Input: part model. Units: mm. Frame: model coordinates. A direction names the side the tool comes from. Give positions to 0.01 mm unless a question says otherwise; leave off trailing zeros. Loops run counter-clockwise (first coordinate to the right, second up) from the corner with the lowest first, then second, coordinate; pieces in that order, holes last. Notation, with made-up numbers: M 89,35.25 L 118,35.25 A25 cw 118,55.25 Z; hole C 89.5,46.5 d11. An arc over 180 degrees is marked long. One line per item, written item: value. Start each with the question number.
(1) Section A-A on y = 1.85. State how many separate pieces and enclosed holes the cut face has, plus the area to 3 significant figures.
(2) Access query for faces 1 (the cylindrical face through (-1.2, 1.5, -8.6)), 2 (the flat face through (66.183, 1.479, 16.42)). Directions: +Z, -Z, +X, -X, +Y, -Y. A direction counts if a zero-diameter tool reaches every point of the face in a straight line with its end or side. Return the directions, or none.
(3) Ray query, line 1 along X through (y, z) = (1.9, 18); line 2 along X through (y, z) = (2, -3); line 3 along Z through (x, y) = (47, 1). Return the intervals inside material, ascending. Write a range as from..to.
(4) Pull-direction query (X, two-part tool) for faces 3 (the flat face through (-94, 1.5, 16.2)), 4 (the flat face through (93.85, 1.48, 16.38)), 5 (the cylindrical face through (-85.414, 1.521, -7.208)), 6 (the flat face through (-1, 3, -5)); classes: released by +X, released by -X, zero draft, split by the parting line, or undercut.
(5) Section B-B on x = -38. Output: boundary loops of the cut face in (y, z), plus the area to 3 significant figures.
```python
from build123d import *

# Parameters (mm, degrees)
SKETCH_1_W             = 200
SKETCH_1_H             = 48
EXTRUDE_1_DEPTH        = 3
SKETCH_2_R             = 2
CUT_EXTRUDE_1_DEPTH    = 3
SKETCH_3_R             = 10.5
CUT_EXTRUDE_2_DEPTH    = 0.1
SKETCH_5_R             = 2
SKETCH_5_R_2           = 1.6
CUT_EXTRUDE_3_DEPTH    = 10
SKETCH_7_W             = 200
SKETCH_7_H             = 1.5
CUT_EXTRUDE_4_DEPTH    = 10
SKETCH_9_R             = 10.5
SKETCH_9_R_2           = 1.6
SKETCH_9_R_3           = 2
EXTRUDE_3_DEPTH        = 0.1
CUT_EXTRUDE_3602_DEPTH = 10
SKETCH_11_W            = 11
SKETCH_11_H            = 7
CUT_EXTRUDE_6_DEPTH    = 10
FILLET_1_R             = 5
FILLET_2_R             = 5
FILLET_3_R             = 0.8


with BuildPart() as part:
    # 草图1 → 凸台-拉伸1 (new body)
    with BuildSketch(Plane(origin=(0, 0, 0), x_dir=(1, 0, 0), z_dir=(0, 1, 0))):
        Rectangle(SKETCH_1_W, SKETCH_1_H)
    extrude(amount=EXTRUDE_1_DEPTH)

    # 草图2 → 切除-拉伸1 (cut)
    with BuildSketch(Plane(origin=(0, 3, 0), x_dir=(1, 0, 0), z_dir=(0, 1, 0))):
        with Locations(Location((-80, -18, 0), (0, 0, 270))):
            Circle(SKETCH_2_R)
        with Locations(Location((0, -18, 0), (0, 0, 270))):
            Circle(SKETCH_2_R)
        with Locations(Location((80, -18, 0), (0, 0, 90))):
            Circle(SKETCH_2_R)
        with Locations(Location((-30, 15, 0), (0, 0, 270))):
            Circle(SKETCH_2_R)
        with Locations(Location((50, 15, 0), (0, 0, 270))):
            Circle(SKETCH_2_R)
    extrude(amount=-CUT_EXTRUDE_1_DEPTH, mode=Mode.SUBTRACT)

    # 草图3 → 切除-拉伸2 (cut)
    with BuildSketch(Plane(origin=(0, 3, 0), x_dir=(1, 0, 0), z_dir=(0, 1, 0))):
        with Locations(Location((-80, 7, 0), (0, 0, 270))):
            Circle(SKETCH_3_R)
        with Locations(Location((0, 7, 0), (0, 0, 270))):
            Circle(SKETCH_3_R)
        with Locations(Location((80, 7, 0), (0, 0, 90))):
            Circle(SKETCH_3_R)
    extrude(amount=-CUT_EXTRUDE_2_DEPTH, mode=Mode.SUBTRACT)

    # 草图5 → 切除-拉伸3 (cut)
    with BuildSketch(Plane(origin=(0, 3, 0), x_dir=(1, 0, 0), z_dir=(0, 1, 0))):
        with Locations(Location((0, 7, 0), (0, 0, 270))):
            Circle(SKETCH_5_R)
        with Locations(Location((0, 14, 0), (0, 0, 270))):
            Circle(SKETCH_5_R_2)
        with Locations(Location((-7, 7, 0), (0, 0, 270))):
            Circle(SKETCH_5_R_2)
        with Locations(Location((7, 7, 0), (0, 0, 270))):
            Circle(SKETCH_5_R_2)
        with Locations(Location((0, 0, 0), (0, 0, 270))):
            Circle(SKETCH_5_R_2)
        with Locations(Location((-80, 0, 0), (0, 0, 270))):
            Circle(SKETCH_5_R_2)
        with Locations(Location((-87, 7, 0), (0, 0, 270))):
            Circle(SKETCH_5_R_2)
        with Locations(Location((-73, 7, 0), (0, 0, 270))):
            Circle(SKETCH_5_R_2)
        with Locations(Location((-80, 14, 0), (0, 0, 270))):
            Circle(SKETCH_5_R_2)
        with Locations(Location((-80, 7, 0), (0, 0, 270))):
            Circle(SKETCH_5_R)
        with Locations(Location((80, 7, 0), (0, 0, 90))):
            Circle(SKETCH_5_R)
        with Locations(Location((80, 14, 0), (0, 0, 90))):
            Circle(SKETCH_5_R_2)
        with Locations(Location((73, 7, 0), (0, 0, 90))):
            Circle(SKETCH_5_R_2)
        with Locations(Location((87, 7, 0), (0, 0, 90))):
            Circle(SKETCH_5_R_2)
        with Locations(Location((80, 0, 0), (0, 0, 90))):
            Circle(SKETCH_5_R_2)
    extrude(amount=-CUT_EXTRUDE_3_DEPTH, mode=Mode.SUBTRACT)

    # 草图7 → 切除-拉伸4 (cut)
    with BuildSketch(Plane(origin=(0, 3, 0), x_dir=(1, 0, 0), z_dir=(0, 1, 0))):
        with Locations((0, 23.25)):
            Rectangle(SKETCH_7_W, SKETCH_7_H)
    extrude(amount=-CUT_EXTRUDE_4_DEPTH, mode=Mode.SUBTRACT)

    # 草图9 → 凸台-拉伸3 (add)
    # profile 1 of 3: a face of its own
    with BuildSketch(Plane(origin=(0, 3, 0), x_dir=(1, 0, 0), z_dir=(0, 1, 0))):
        with Locations((80, 7)):
            Circle(SKETCH_9_R)
        with Locations(Location((73, 7, 0), (0, 0, 270))):
            Circle(SKETCH_9_R_2, mode=Mode.SUBTRACT)
        with Locations(Location((80, 14, 0), (0, 0, 270))):
            Circle(SKETCH_9_R_2, mode=Mode.SUBTRACT)
        with Locations(Location((80, 7, 0), (0, 0, 270))):
            Circle(SKETCH_9_R_3, mode=Mode.SUBTRACT)
        with Locations(Location((87, 7, 0), (0, 0, 270))):
            Circle(SKETCH_9_R_2, mode=Mode.SUBTRACT)
        with Locations(Location((80, 0, 0), (0, 0, 270))):
            Circle(SKETCH_9_R_2, mode=Mode.SUBTRACT)
    # profile 2 of 3: a face of its own
    with BuildSketch(Plane(origin=(0, 3, 0), x_dir=(1, 0, 0), z_dir=(0, 1, 0))):
        with Locations((0, 7)):
            Circle(SKETCH_9_R)
        with Locations(Location((0, 7, 0), (0, 0, 270))):
            Circle(SKETCH_9_R_3, mode=Mode.SUBTRACT)
        with Locations(Location((0, 14, 0), (0, 0, 270))):
            Circle(SKETCH_9_R_2, mode=Mode.SUBTRACT)
        with Locations(Location((-7, 7, 0), (0, 0, 270))):
            Circle(SKETCH_9_R_2, mode=Mode.SUBTRACT)
        with Locations(Location((7, 7, 0), (0, 0, 270))):
            Circle(SKETCH_9_R_2, mode=Mode.SUBTRACT)
        with Locations(Location((0, 0, 0), (0, 0, 270))):
            Circle(SKETCH_9_R_2, mode=Mode.SUBTRACT)
    # profile 3 of 3: a face of its own
    with BuildSketch(Plane(origin=(0, 3, 0), x_dir=(1, 0, 0), z_dir=(0, 1, 0))):
        with Locations((-80, 7)):
            Circle(SKETCH_9_R)
        with Locations(Location((-87, 7, 0), (0, 0, 270))):
            Circle(SKETCH_9_R_2, mode=Mode.SUBTRACT)
        with Locations(Location((-80, 0, 0), (0, 0, 270))):
            Circle(SKETCH_9_R_2, mode=Mode.SUBTRACT)
        with Locations(Location((-80, 14, 0), (0, 0, 270))):
            Circle(SKETCH_9_R_2, mode=Mode.SUBTRACT)
        with Locations(Location((-73, 7, 0), (0, 0, 270))):
            Circle(SKETCH_9_R_2, mode=Mode.SUBTRACT)
        with Locations(Location((-80, 7, 0), (0, 0, 270))):
            Circle(SKETCH_9_R_3, mode=Mode.SUBTRACT)
    extrude(amount=-EXTRUDE_3_DEPTH)

    # 草图10 → Cut-Extrude 3602 (cut)
    with BuildSketch(Plane.XZ):
        Polygon((-100, 9), (-87.5, 24), (-100, 24), align=None)
        Polygon((-72.5, 24), (-7.5, 24), (-20, 9), (-59.913505532, 9), align=None)
        Polygon((72.5, 24), (7.5, 24), (20.086494468, 9), (60, 9), align=None)
        Polygon((87.5, 24), (100, 9), (100, 24), align=None)
    extrude(amount=-CUT_EXTRUDE_3602_DEPTH, mode=Mode.SUBTRACT)

    # 草图11 → 切除-拉伸6 (cut)
    with BuildSketch(Plane.XZ):
        with Locations((-54.5, 0)):
            Rectangle(SKETCH_11_W, SKETCH_11_H)
        with Locations((21.5, 0)):
            Rectangle(SKETCH_11_W, SKETCH_11_H)
        with Locations((54.5, 0)):
            Rectangle(SKETCH_11_W, SKETCH_11_H)
    extrude(amount=-CUT_EXTRUDE_6_DEPTH, mode=Mode.SUBTRACT)

    # 圆角1
    fillet_1_edges = [part.edges().sort_by_distance(p)[0] for p in [
        (100, 1.5, -22.5),
        (-100, 1.5, -22.5),
    ]]
    fillet(fillet_1_edges, radius=FILLET_1_R)

    # 圆角2
    fillet_2_edges = [part.edges().sort_by_distance(p)[0] for p in [
        (-100, 1.5, 9),
        (-87.5, 1.5, 24),
        (-7.5, 1.5, 24),
        (-20, 1.5, 9),
        (-59.913505532, 1.5, 9),
        (-72.5, 1.5, 24),
        (20.086494468, 1.5, 9),
        (7.5, 1.5, 24),
        (72.5, 1.5, 24),
        (60, 1.5, 9),
        (87.5, 1.5, 24),
        (100, 1.5, 9),
    ]]
    fillet(fillet_2_edges, radius=FILLET_2_R)

    # 圆角3
    fillet_3_edges = [part.edges().sort_by_distance(p)[0] for p in [
        (-60, 1.5, -3.5),
        (-60, 1.5, 3.5),
        (-49, 1.5, 3.5),
        (-49, 1.5, -3.5),
        (16, 1.5, -3.5),
        (16, 1.5, 3.5),
        (27, 1.5, 3.5),
        (27, 1.5, -3.5),
        (49, 1.5, -3.5),
        (49, 1.5, 3.5),
        (60, 1.5, 3.5),
        (60, 1.5, -3.5),
    ]]
    fillet(fillet_3_edges, radius=FILLET_3_R)


solid = part.part
```
Output values:
1. separate pieces: 1
1. enclosed holes: 23
1. area: 7,100 mm²
2. face 1: +Y, -Y
2. face 2: +Z, +Y, -Y
3. line 1: x = -92.5..-82, -78..-67.47, -12.5..-2, 2..12.53, 67.5..78, 82..92.5
3. line 2: x = -100..-59.94, -49.06..16.06, 26.94..49.06, 59.94..100
3. line 3: z = -22.5..9
4. face 3: released by -X
4. face 4: released by +X
4. face 5: undercut
4. face 6: zero draft
5. outline: M 0,-22.5 L 3,-22.5 L 3,9 L 0,9 Z
5. area: 94.5 mm²
